from build123d import *

# Parameters (mm, degrees)
BOSS_EXTRUDE1_DEPTH = 50.8
SKETCH6_R           = 9.525
CUT_EXTRUDE1_DEPTH  = 50.8
SKETCH7_R           = 25.4
CUT_EXTRUDE2_DEPTH  = 17.526
SKETCH8_R           = 6.35
CUT_EXTRUDE3_DEPTH  = 26.4
SKETCH9_R           = 6.35
CUT_EXTRUDE4_DEPTH  = 26.4


with BuildPart() as part:
    # Sketch5 → Boss-Extrude1 (new body)
    with BuildSketch(Plane.XY):
        with BuildLine():
            Line((6.35, 25.4), (57.15, 25.4))
            ThreePointArc((57.15, 25.4), (61.640128061, 27.259871939), (63.5, 31.75))
            Line((63.5, 31.75), (63.5, 97.24338288))
            ThreePointArc((63.5, 97.24338288), (65.359871939, 101.73351094), (69.85, 103.59338288))
            Line((69.85, 103.59338288), (133.35, 103.59338288))
            ThreePointArc((133.35, 103.59338288), (137.840128061, 101.73351094), (139.7, 97.24338288))
            Line((139.7, 97.24338288), (139.7, 31.75))
            ThreePointArc((139.7, 31.75), (141.559871939, 27.259871939), (146.05, 25.4))
            Line((146.05, 25.4), (196.85, 25.4))
            ThreePointArc((196.85, 25.4), (201.340128061, 23.540128061), (203.2, 19.05))
            Line((203.2, 19.05), (203.2, 0))
            Line((203.2, 0), (152.4, 0))
            Line((152.4, 0), (152.4, 7.62))
            Line((152.4, 7.62), (50.8, 7.62))
            Line((50.8, 7.62), (50.8, 0))
            Line((50.8, 0), (0, 0))
            Line((0, 0), (0, 19.05))
            ThreePointArc((0, 19.05), (1.859871939, 23.540128061), (6.35, 25.4))
        make_face()
    extrude(amount=-BOSS_EXTRUDE1_DEPTH)

    # Sketch6 → Cut-Extrude1 (cut)
    with BuildSketch(Plane.XY):
        with Locations((101.6, 63.5)):
            Circle(SKETCH6_R)
    extrude(amount=-CUT_EXTRUDE1_DEPTH, mode=Mode.SUBTRACT)

    # Sketch7 → Cut-Extrude2 (cut)
    with BuildSketch(Plane.XY):
        with Locations((101.6, 63.5)):
            Circle(SKETCH7_R)
    extrude(amount=-CUT_EXTRUDE2_DEPTH, mode=Mode.SUBTRACT)

    # Sketch8 → Cut-Extrude3 (cut, through all)
    with BuildSketch(Plane(origin=(0, 25.4, 0), x_dir=(1, 0, 0), z_dir=(0, 1, 0))):
        with Locations((25.4, 25.4)):
            Circle(SKETCH8_R)
    extrude(amount=-CUT_EXTRUDE3_DEPTH, mode=Mode.SUBTRACT)

    # Sketch9 → Cut-Extrude4 (cut, through all)
    with BuildSketch(Plane(origin=(0, 25.4, 0), x_dir=(1, 0, 0), z_dir=(0, 1, 0))):
        with Locations((177.8, 25.4)):
            Circle(SKETCH9_R)
    extrude(amount=-CUT_EXTRUDE4_DEPTH, mode=Mode.SUBTRACT)


solid = part.part
For this review, take the finished solid that the model builds, in its own axes (mm). A direction names the side the tool comes from. Round coordinates to 2 decimals unless told otherwise and drop trailing zeros. Loops run counter-clockwise (first coordinate to the right, second up) from the corner with the lowest first, then second, coordinate; pieces in that order, holes last. Notation, with made-up numbers: (-22.5, 72) - (-14.5, 72) arc R10 cw to (-14.5, 91) - close; hole circle Ø4 at (49, 87.5). An arc over 180 degrees is marked (long way). Use one line per item in the form item = value.
Item 1: Consider section C-C on y = 63.5. Write out the cut boundary in (x, z) (3 decimals).
Answers:
outline = (63.5, -50.8) - (92.075, -50.8) - (92.075, -17.526) - (76.2, -17.526) - (76.2, 0) - (63.5, 0) - close; (111.125, -50.8) - (139.7, -50.8) - (139.7, 0) - (127, 0) - (127, -17.526) - (111.125, -17.526) - close
Item 2: For line 1 (X direction, y = 14.75, z = -25.4); line 2 (X direction, y = 21, z = -20.5); line 3 (Y direction, x = 101, z = -8), list the stretches that pass through material, from the lowest coordinate up.
Answers:
line_1 = 0 to 19.05, 31.75 to 171.45, 184.15 to 203.2
line_2 = 0.31 to 21.36, 29.44 to 173.76, 181.84 to 202.89
line_3 = 7.62 to 38.11, 88.89 to 103.59
Item 3: Consider section B-B on x = 101.6. Write out the cut boundary in (y, z) (3 decimals), then the cut area to 3 significant figures.
Answers:
outline = (7.62, -50.8) - (53.975, -50.8) - (53.975, -17.526) - (38.1, -17.526) - (38.1, 0) - (7.62, 0) - close; (73.025, -50.8) - (103.593, -50.8) - (103.593, 0) - (88.9, 0) - (88.9, -17.526) - (73.025, -17.526) - close
area = 3,350 mm^2
Item 4: Consider section A-A on z = -25.4. Write out the cut boundary in (x, y) (3 decimals), then the cut area to 3 significant figures.
Answers:
outline = (0, 0) - (19.05, 0) - (19.05, 25.4) - (6.35, 25.4) arc R6.35 ccw to (0, 19.05) - close; (31.75, 0) - (50.8, 0) - (50.8, 7.62) - (152.4, 7.62) - (152.4, 0) - (171.45, 0) - (171.45, 25.4) - (146.05, 25.4) arc R6.35 cw to (139.7, 31.75) - (139.7, 97.243) arc R6.35 ccw to (133.35, 103.593) - (69.85, 103.593) arc R6.35 ccw to (63.5, 97.243) - (63.5, 31.75) arc R6.35 cw to (57.15, 25.4) - (31.75, 25.4) - close; (184.15, 0) - (203.2, 0) - (203.2, 19.05) arc R6.35 ccw to (196.85, 25.4) - (184.15, 25.4) - close; hole circle Ø19.05 at (101.6, 63.5)
area = 9,400 mm^2
Item 5: Mouldability with a two-part tool opening along X and no side actions: class faces 4 (the cylindrical face through (172.76, 12.88, -21.54)), 5 (the flat face through (0, 9, -25)), 6 (the flat face through (171, 25.4, -25)), 7 (the flat face through (102, 7.62, -25)) as +X half, -X half, draft (parallel to the pull), parting line (faces both ways), or undercut.
Answers:
face_4 = undercut
face_5 = -X half
face_6 = draft
face_7 = undercut
Item 6: Clearance check with flat-ended pins moving along their axes: P1, Ø1.5, axis at y = 89, z = -45.5, coming from the +X side; P2, Ø15, axis at x = 174, z = -16, coming from the +Y side; P3, Ø7.5, axis at x = 25.4, z = -25.4, coming from the -Y side; P4, Ø15, axis at x = 109.5, y = 66.5, coming from the +Z side. State where each tip first meets the part, or that it passes through.
Answers:
P1 = 139.7
P2 = 25.4
P3 = through
P4 = -17.53
Item 7: Consider section D-D on z = -45. Write out the cut boundary in (x, y) (3 decimals).
Answers:
outline = (0, 0) - (50.8, 0) - (50.8, 7.62) - (152.4, 7.62) - (152.4, 0) - (203.2, 0) - (203.2, 19.05) arc R6.35 ccw to (196.85, 25.4) - (146.05, 25.4) arc R6.35 cw to (139.7, 31.75) - (139.7, 97.243) arc R6.35 ccw to (133.35, 103.593) - (69.85, 103.593) arc R6.35 ccw to (63.5, 97.243) - (63.5, 31.75) arc R6.35 cw to (57.15, 25.4) - (6.35, 25.4) arc R6.35 ccw to (0, 19.05) - close; hole circle Ø19.05 at (101.6, 63.5)
Item 8: Tool access review of faces 1 (the flat face through (139.7, 65, -25)), 2 (the flat face through (37, 25.4, -25)), 3 (the flat face through (113, 64, -17.526)): name each direction out of +Z, -Z, +X, -X, +Y, -Y from which nothing blocks a thin tool from reaching the whole face with its end or side.
Answers:
face_1 = +Z, -Z, +X, +Y
face_2 = +Z, -Z, -X, +Y
face_3 = +Z
